Geometry: final body of the model. Coordinates: model frame, mm. A direction names the side the tool comes from. Give positions to 0.01 mm unless a question says otherwise; leave off trailing zeros. Loops run counter-clockwise (first coordinate to the right, second up) from the corner with the lowest first, then second, coordinate; pieces in that order, holes last. Notation, with made-up numbers: (2.25, 76.5) -> (51.25, 76.5) arc R22 ccw to (51.25, 89.5) -> close; hole circle Ø11 at (-30.5, 44). An arc over 180 degrees is marked (long way). Answer in a Markdown table with one row per item. Add a question column.
from build123d import *

# Parameters (mm, degrees)
SM_BASE_FLANGE_1_DEPTH           = 22
FILLET_1_R                       = 3
HOLE_WIZARD_6_8_6_8_1_DEPTH      = 1
HOLE_WIZARD_3_1_3_1_1_AT_2_COUNT = 2
HOLE_WIZARD_3_1_3_1_1_AT_2_PITCH = 41.340053217
HOLE_WIZARD_3_1_3_1_1_AT_3_COUNT = 2
HOLE_WIZARD_3_1_3_1_1_AT_3_PITCH = 22
HOLE_WIZARD_3_1_3_1_1_AT_4_COUNT = 2
HOLE_WIZARD_3_1_3_1_1_AT_4_PITCH = 35


# Read off the part's stored shape, not the designer's step: Диаметр отверстия Ø6.8 (6.8)1
# Sheet-metal steps are written as plain solids
with BuildPart() as part:
    # Sketch 1 → Базовая кромка1 (new, symmetric)
    with BuildSketch(Plane(origin=(0, 0, 0), x_dir=(1, 0, 0), z_dir=(0, 1, 0))):
        with BuildLine():
            Line((0, -21.5), (0, -2))
            ThreePointArc((0, -2), (0.585786438, -0.585786438), (2, 0))
            Line((2, 0), (50, 0))
            Line((50, 0), (50, -1))
            Line((50, -1), (2, -1))
            ThreePointArc((2, -1), (1.292893219, -1.292893219), (1, -2))
            Line((1, -2), (1, -21.5))
            Line((1, -21.5), (0, -21.5))
        make_face()
    extrude(amount=SM_BASE_FLANGE_1_DEPTH, both=True)

    # Скругление1
    fillet_1_edges = [part.edges().sort_by_distance(p)[0] for p in [
        (0.5, 22, 21.5),
        (0.5, -22, 21.5),
        (50, 22, 0.5),
        (50, -22, 0.5),
    ]]
    fillet(fillet_1_edges, radius=FILLET_1_R)

    # Диаметр отверстия Ø6.8 (6.8)1 outline → Диаметр отверстия Ø6.8 (6.8)1 (cut)
    with BuildSketch(Plane.YZ):
        with BuildLine():
            Line((-12.375, 10.25), (-12.375, 13.75))
            ThreePointArc((-12.375, 13.75), (-15.875, 17.25), (-19.375, 13.75))
            Line((-19.375, 13.75), (-19.375, 10.25))
            ThreePointArc((-19.375, 10.25), (-15.875, 6.75), (-12.375, 10.25))
        make_face()
        with BuildLine():
            ThreePointArc((19.375, 13.75), (15.875, 17.25), (12.375, 13.75))
            Line((12.375, 13.75), (12.375, 10.25))
            ThreePointArc((12.375, 10.25), (15.875, 6.75), (19.375, 10.25))
            Line((19.375, 10.25), (19.375, 13.75))
        make_face()
    extrude(amount=HOLE_WIZARD_6_8_6_8_1_DEPTH, mode=Mode.SUBTRACT)

    # Эскиз5 → Диаметр отверстия Ø3.1 (3.1)1 (revolve, cut)
    with BuildSketch(Plane(origin=(6.5, 9, 1), x_dir=(0, -1, 0), z_dir=(1, 0, 0))):
        Polygon((0, 0), (0, 1), (1.55, 1), (1.55, 0.7), (2.25, 0), align=None)
    hole_wizard_3_1_3_1_1 = revolve(axis=Axis((6.5, 9, 7.35), (0, 0, -1)), mode=Mode.SUBTRACT)

    # Диаметр отверстия Ø3.1 (3.1)1 at 2: Диаметр отверстия Ø3.1 (3.1)1 ×2
    with Locations(*[Vector(0.8466365492110047, -0.5321715452183459, 0) * (i * HOLE_WIZARD_3_1_3_1_1_AT_2_PITCH) for i in range(1, HOLE_WIZARD_3_1_3_1_1_AT_2_COUNT)]):
        add(hole_wizard_3_1_3_1_1, mode=Mode.SUBTRACT)

    # Диаметр отверстия Ø3.1 (3.1)1 at 3: Диаметр отверстия Ø3.1 (3.1)1 ×2
    with Locations(*[(0, -i * HOLE_WIZARD_3_1_3_1_1_AT_3_PITCH, 0) for i in range(1, HOLE_WIZARD_3_1_3_1_1_AT_3_COUNT)]):
        add(hole_wizard_3_1_3_1_1, mode=Mode.SUBTRACT)

    # Диаметр отверстия Ø3.1 (3.1)1 at 4: Диаметр отверстия Ø3.1 (3.1)1 ×2
    with Locations(*[(i * HOLE_WIZARD_3_1_3_1_1_AT_4_PITCH, 0, 0) for i in range(1, HOLE_WIZARD_3_1_3_1_1_AT_4_COUNT)]):
        add(hole_wizard_3_1_3_1_1, mode=Mode.SUBTRACT)


solid = part.part
(1) Cut plane B-B on y = 9. Return the cut outline in (x, z).
(2) Pin query (flat end, axial travel): pin 1 Ø2 at (y, z) = (-10, 3) entering from +X; pin 2 Ø12 at (x, y) = (41, -8) entering from +Z; pin 3 Ø4 at (x, y) = (6.5, 9) entering from +Z. Return the tip coordinate at first contact, or that it passes through.
(3) Cut plane D-D on y = -13. Return the cut outline in (x, z), then the cut area to 3 significant figures.
(4) Reachability of faces 4 (the cylindrical face through (0.49, -15.95, 6.75)), 5 (the flat face through (26, 0, 1)), 6 (the cylindrical face through (0.57, 0.31, 0.6)) from +Z, -Z, +X, -X, +Y, -Y: full face, straight path, thin tool, end or side. Return the list, or none.
(5) Cut plane A-A on z = 11.75. Return the cut outline in (x, y) (3 decimals).
(6) Material intervals for line 1 along Y through (x, z) = (41.5, 0.2); line 2 along X through (y, z) = (-13, 0.25); line 3 along X through (y, z) = (18, 4.5), sorted ascending. Write a range as from..to.
(7) Draft query along Y for faces 1 (the cylindrical face through (0.49, 21.14, 20.6)), 2 (the cylindrical face through (0.49, -21.14, 20.6)), 3 (the cylindrical face through (0.49, 15.8, 6.75)). Return one class per face: +Y half, -Y half, draft (parallel to the pull), parting line (faces both ways), or undercut.
(8) Cut plane C-C on x = 6.5. Return the cut outline in (y, z).
Answer list:
| question | item | result |
|---|---|---|
| 1 | outline | (0, 2) arc R2 ccw to (2, 0) -> (4.95, 0) -> (4.95, 0.3) -> (4.25, 1) -> (2, 1) arc R1 cw to (1, 2) -> (1, 21.5) -> (0, 21.5) -> close; (8.05, 0) -> (39.95, 0) -> (39.95, 0.3) -> (39.25, 1) -> (8.75, 1) -> (8.05, 0.3) -> close; (43.05, 0) -> (50, 0) -> (50, 1) -> (43.75, 1) -> (43.05, 0.3) -> close |
| 2 | pin 1 | stops at x = 1 |
| 2 | pin 2 | stops at z = 1 |
| 2 | pin 3 | stops at z = 0.75 |
| 3 | outline | (0, 2) arc R2 ccw to (2, 0) -> (4.95, 0) -> (4.95, 0.3) -> (4.25, 1) -> (2, 1) arc R1 cw to (1, 2) -> (1, 8.25) -> (0, 8.25) -> close; (0, 15.75) -> (1, 15.75) -> (1, 21.5) -> (0, 21.5) -> close; (8.05, 0) -> (39.95, 0) -> (39.95, 0.3) -> (39.25, 1) -> (8.75, 1) -> (8.05, 0.3) -> close; (43.05, 0) -> (50, 0) -> (50, 1) -> (43.75, 1) -> (43.05, 0.3) -> close |
| 3 | area | 55.2 mm² |
| 4 | face 4 | +X, -X |
| 4 | face 5 | +Z, +X, +Y, -Y |
| 4 | face 6 | -Z, -X, +Y, -Y |
| 5 | outline | (0, -22) -> (1, -22) -> (1, -19.375) -> (0, -19.375) -> close; (0, -12.375) -> (1, -12.375) -> (1, 12.375) -> (0, 12.375) -> close; (0, 19.375) -> (1, 19.375) -> (1, 22) -> (0, 22) -> close |
| 6 | line 1 | y = -22..-14.55, -11.45..7.45, 10.55..22 |
| 6 | line 2 | x = 1.03..4.95, 8.05..39.95, 43.05..50 |
| 6 | line 3 | x = 0..1 |
| 7 | face 1 | +Y half |
| 7 | face 2 | -Y half |
| 7 | face 3 | undercut |
| 8 | outline | (-22, 0) -> (-14.55, 0) -> (-14.55, 0.3) -> (-15.25, 1) -> (-22, 1) -> close; (-11.45, 0) -> (7.45, 0) -> (7.45, 0.3) -> (6.75, 1) -> (-10.75, 1) -> (-11.45, 0.3) -> close; (10.55, 0) -> (22, 0) -> (22, 1) -> (11.25, 1) -> (10.55, 0.3) -> close |
